Source: CAD feature listing. Evaluate the final solid. Frame: model axes, mm. A direction names the side the tool comes from. Give positions to 0.01 mm unless a question says otherwise; leave off trailing zeros. Loops run counter-clockwise (first coordinate to the right, second up) from the corner with the lowest first, then second, coordinate; pieces in that order, holes last.
```python
from build123d import *

# Parameters (mm, degrees)
F0_W     = 50.8
F0_H     = 50.8
F0_W_2   = 25.4
F0_H_2   = 25.4
F1_DEPTH = 88.9
F2_W     = 56.879024
F2_H     = 39.945584
F3_DEPTH = 50.8


with BuildPart() as f1:
    # F0 (on Right) → F1 (new body)
    with BuildSketch(Plane.YZ):
        with Locations((-2.20958, 0)):
            Rectangle(F0_W, F0_H)
        with Locations((-2.20958, 0)):
            Rectangle(F0_W_2, F0_H_2, mode=Mode.SUBTRACT)
    extrude(amount=F1_DEPTH)

    # F2 (on face) → F3 (cut)
    with BuildSketch(Plane.XZ.offset(27.60958)):
        with Locations((44.750276, 5.427208)):
            Rectangle(F2_W, F2_H)
    extrude(amount=-F3_DEPTH, mode=Mode.SUBTRACT)


solid = f1.part
```
(1) Section D-D, the plane z = 3.5. Return the cut outline in (x, y).
A:
outline: (0, -27.61) - (16.31, -27.61) - (16.31, -14.91) - (0, -14.91) - close; (0, 10.49) - (16.31, 10.49) - (16.31, 23.19) - (0, 23.19) - close; (73.19, -27.61) - (88.9, -27.61) - (88.9, -14.91) - (73.19, -14.91) - close; (73.19, 10.49) - (88.9, 10.49) - (88.9, 23.19) - (73.19, 23.19) - close
(2) Section A-A, the plane y = -6. Return the cut outline in (x, z).
A:
outline: (0, -25.4) - (88.9, -25.4) - (88.9, -12.7) - (73.19, -12.7) - (73.19, -14.55) - (16.31, -14.55) - (16.31, -12.7) - (0, -12.7) - close; (0, 12.7) - (16.31, 12.7) - (16.31, 25.4) - (0, 25.4) - close; (73.19, 12.7) - (88.9, 12.7) - (88.9, 25.4) - (73.19, 25.4) - close
(3) Section C-C, the plane z = 15.5. Return the cut outline in (x, y).
A:
outline: (0, -27.61) - (16.31, -27.61) - (16.31, 23.19) - (0, 23.19) - close; (73.19, -27.61) - (88.9, -27.61) - (88.9, 23.19) - (73.19, 23.19) - close
(4) Mould query, pull axis X, two halves, no side actions, for faces 4 (the flat face through (88.9, -3, 17)), 5 (the flat face through (73.19, -3, 14)), 6 (the flat face through (81, -2, 12.7)), 7 (the flat face through (0, -3, 17)). Classes: pulls with the +X half, pulls with the -X half, needs draft (parallel to the pull), parting line crosses it, or undercut.
A:
face 4: pulls with the +X half
face 5: undercut
face 6: needs draft
face 7: pulls with the -X half
(5) Ray query, line 1 along X through (y, z) = (17.5, 2.5); line 2 along Z through (x, y) = (77, -10); line 3 along Y through (x, z) = (82, -6). Return the intervals inside material, ascending.
A:
line 1: x = 0 to 16.31, 73.19 to 88.9
line 2: z = -25.4 to -12.7, 12.7 to 25.4
line 3: y = -27.61 to -14.91, 10.49 to 23.19
(6) Reachability of faces 1 (the flat face through (8, -2, -12.7)), 2 (the flat face through (44, -3, -14.546)), 3 (the flat face through (8, -3, 25.4)) from +Z, -Z, +X, -X, +Y, -Y: full face, straight path, thin tool, end or side. Return the list, or none.
A:
face 1: +X, -X
face 2: +Z, +Y, -Y
face 3: +Z, +X, -X, +Y, -Y
(7) Section B-B, the plane x = 82. Return the cut outline in (y, z), then the cut area to 3 significant figures.
A:
outline: (-27.61, -25.4) - (23.19, -25.4) - (23.19, 25.4) - (-27.61, 25.4) - close; hole (-14.91, -12.7) - (10.49, -12.7) - (10.49, 12.7) - (-14.91, 12.7) - close
area: 1,940 mm2
(8) First-contact query: pin 1 (8 mm diameter, centred on x = 37, y = -19.5, fed in from +Z). Flat tip, straight axial feed; report the tip coordinate or a pass-through.
A:
pin 1: stops at z = -14.55
